Can you work these out from the model? Positions are in its coordinate system, mm. Face numbers are marked on the shaded views. A direction names the side the tool comes from. Give positions to 0.01 mm unless a question says otherwise; leave off trailing zeros. Loops run counter-clockwise (first coordinate to the right, second up) from the corner with the lowest first, then second, coordinate; pieces in that order, holes last. Notation, with made-up numbers: (-37.75, 61.25) - (-7.75, 61.25) arc R37 cw to (-7.75, 97.25) - close; hole circle Ø8 at (85.25, 88). An arc over 180 degrees is marked (long way). Answer as a JSON object with one key per item and string values. Group by question number.
Item 1: Please list where these lines run through material, in increasing order: L1, parallel to X at y = -7.75, z = 10.5; L2, parallel to Z at x = 8, y = -8.5; L3, parallel to X at y = 4, z = 4.25.
Item 2: Thinking about a two-plate mould opening in X: for the marked faces 1, 2 and 3, which applies, pulls with the +X half, pulls with the -X half, needs draft (parallel to the pull), parting line crosses it, or undercut?
Item 3: Suppose I cut it at C-C on x = 13.25. Write out the boundary of the cut face in (y, z).
Item 4: Suppose I cut it at B-B on y = 3. Write out the boundary of the cut face in (x, z), and give its area (3 significant figures).
Item 5: Will these pins go through, and if not, where does the flat tip stop? pin 1 (5 mm diameter, centred on x = 6, y = -5.5, fed in from -Z); pin 2 (4.5 mm diameter, centred on x = 9.36, y = -2.78, fed in from +Z).
Item 6: Which directions (+Z, -Z, +X, -X, +Y, -Y) give clear straight access to the entire face, cutting with the end or side of a thin tool? Please do the marked faces 4 and 5.
Item 7: Suppose I cut it at A-A on z = 15.75. Write out the boundary of the cut face in (x, y).
from build123d import *

# Parameters (mm, degrees)
SZKIC1_W                    = 15
SZKIC1_H                    = 15
DODANIE_WYCI_GNI_CIE2_DEPTH = 23.8
SKORUPA3_T                  = -1.5
ZAOKR_GLENIE1_R             = 1


# Read off the part's stored shape, not the designer's step: Pogłębienie walcowe pod M2 Śrubę z łbem stożkowym ściętym1
with BuildPart() as part:
    # Szkic1 → Dodanie-wyciągnięcie2 (new body)
    with BuildSketch(Plane.XY):
        with Locations((9.359290026, -2.777742542)):
            Rectangle(SZKIC1_W, SZKIC1_H)
    extrude(amount=DODANIE_WYCI_GNI_CIE2_DEPTH)

    # Skorupa3
    skorupa3_openings = [part.faces().sort_by_distance(p)[0] for p in [
        (9.359290026, -2.777742542, 0),
        (9.359290026, -10.277742542, 11.9),
        (9.359290026, 4.722257458, 11.9),
    ]]
    offset(amount=SKORUPA3_T, openings=skorupa3_openings, kind=Kind.INTERSECTION)

    # Zaokrąglenie1
    zaokr_glenie1_edges = [part.edges().sort_by_distance(p)[0] for p in [
        (16.859290026, -10.277742542, 11.9),
        (1.859290026, -10.277742542, 11.9),
        (1.859290026, 4.722257458, 11.9),
        (16.859290026, 4.722257458, 11.9),
    ]]
    fillet(zaokr_glenie1_edges, radius=ZAOKR_GLENIE1_R)

    # Pog_bienie walcowe pod M2 _rub_ z _b 2 → Pogłębienie walcowe pod M2 Śrubę z łbem stożkowym ściętym1 (revolve, cut)
    with BuildSketch(Plane(origin=(9.359290026, -2.777742542, 0), x_dir=(1, 0, 0), z_dir=(0, -1, 0))):
        Polygon((2.525, 23.8), (0, 23.8), (0, 22.3), (2.5, 22.3), (2.5, 23.775), align=None)
    revolve(axis=Axis((9.359290026, -2.777742542, 0), (0, 0, 1)), mode=Mode.SUBTRACT)


solid = part.part
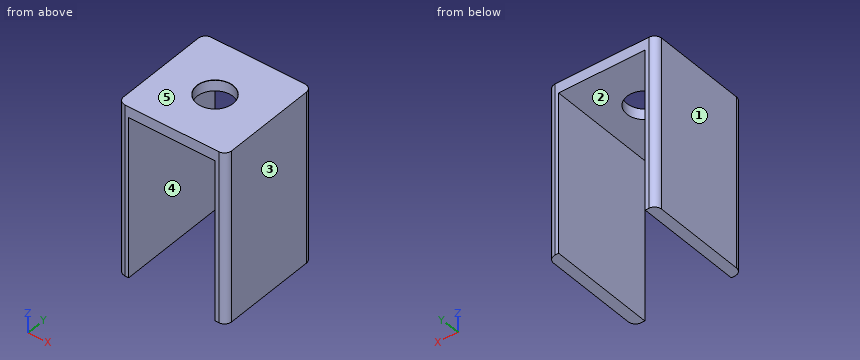
Worked out:
{
 "1": {"L1": "x = 1.86 to 3.36, 15.36 to 16.86", "L2": "z = 22.3 to 23.8", "L3": "x = 1.9 to 3.36, 15.36 to 16.82"},
 "2": {"face 1": "pulls with the -X half", "face 2": "undercut", "face 3": "pulls with the +X half"},
 "3": {"outline": "(-10.28, 22.3) - (4.72, 22.3) - (4.72, 23.8) - (-10.28, 23.8) - close"},
 "4": {"outline": "(1.86, 0) - (3.36, 0) - (3.36, 22.3) - (15.36, 22.3) - (15.36, 0) - (16.86, 0) - (16.86, 23.8) - (1.86, 23.8) - close", "area": "89.4 mm2"},
 "5": {"pin 1": "stops at z = 22.3", "pin 2": "passes through"},
 "6": {"face 4": "-Z, +Y, -Y", "face 5": "+Z, +X, -X, +Y, -Y"},
 "7": {"outline": "(1.86, -9.28) arc R1 ccw to (2.86, -10.28) - (3.36, -10.28) - (3.36, 4.72) - (2.86, 4.72) arc R1 ccw to (1.86, 3.72) - close; (15.36, -10.28) - (15.86, -10.28) arc R1 ccw to (16.86, -9.28) - (16.86, 3.72) arc R1 ccw to (15.86, 4.72) - (15.36, 4.72) - close"}
}
